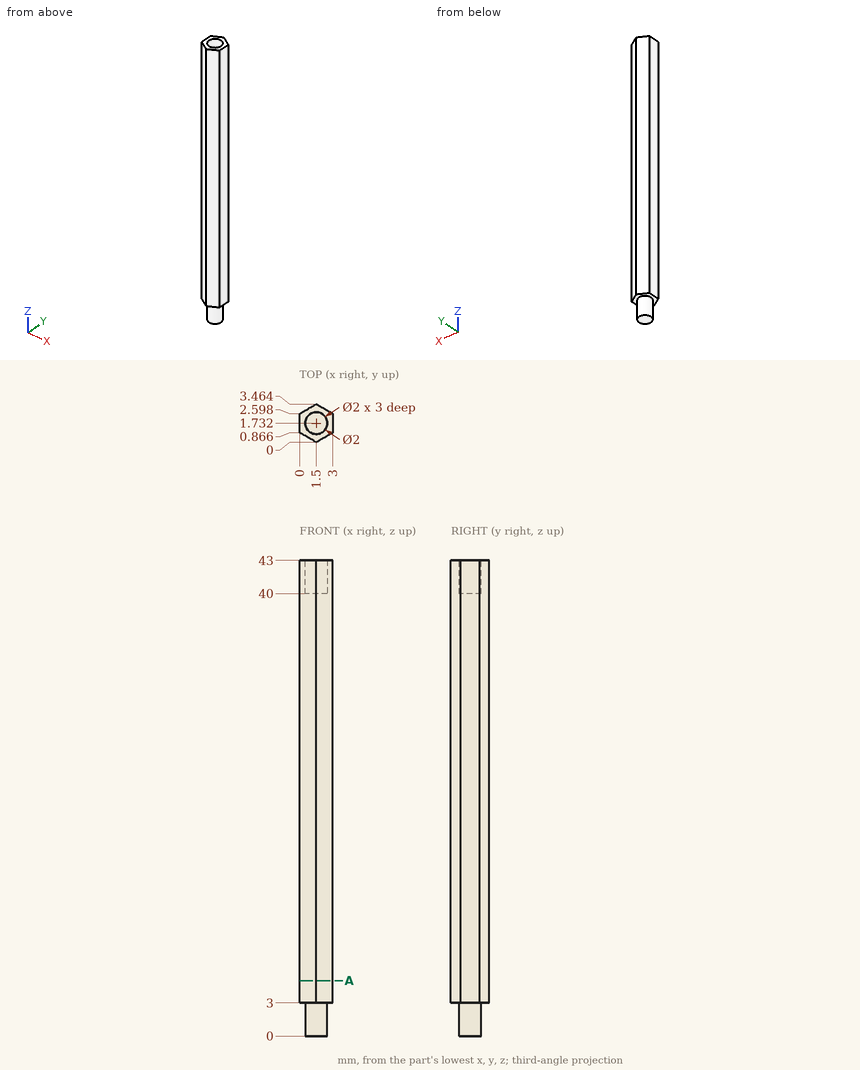
Input: dimensioned drawing with shaded views. Units: mm. Origin: part minimum x, y, z. Coordinates: 2 decimals unless noted, no trailing zeros. Write each loop counter-clockwise with the first axis right and the second up, starting at its lowest first coordinate (ties: lowest second). Pieces come first, ordered by that corner, then holes. Notation, with made-up numbers: M 14.5,-2 L 23.5,-2 A27 cw 23.5,28 Z; hole C 15,-3 d8. An arc over 180 degrees is marked long. Use one line per item in the form item = value.
Q1. Material intervals for probe 1 along Z at (x, y) = (0.35, 2.4); probe 2 along Z at (x, y) = (1.4, 1.85); probe 3 along X at (y, z) = (3.1, 35.5), sorted ascending. Write a range as from..to.
Answer below:
probe_1 = 3..43
probe_2 = 0..40
probe_3 = 0.87..2.13
Q2. First-contact query: pin 1 (1.6 mm diameter, centred on x = 1.5, y = 1.73, fed in from +Z). Flat tip, straight axial feed; report the tip coordinate or a pass-through.
Answer below:
pin_1 = 40
Q3. Section A-A (z = 5). Return loops of the section in (x, y).
Answer below:
outline = M 0,0.87 L 1.5,0 L 3,0.87 L 3,2.6 L 1.5,3.46 L 0,2.6 Z
